```python
from build123d import *

# Parameters (mm, degrees)
BASPROSKE_W     = 100
BASPROSKE_H     = 56
TOOTHCUT_DEPTH  = 128.561749753
TEETHCUTS_COUNT = 12
TEETHCUTS_ANGLE = 330
BORSKE_R        = 20
BORE_DEPTH      = 100.0000508
SCALE1_SCALE    = 0.25


with BuildPart() as part:
    # BasProSke → Base-Revolve (revolve)
    with BuildSketch(Plane(origin=(0, 0, 0), x_dir=(1, 0, 0), z_dir=(0, 1, 0)), mode=Mode.PRIVATE) as base_revolve_sk:
        with Locations((50, 28)):
            Rectangle(BASPROSKE_W, BASPROSKE_H)
    revolve(base_revolve_sk.sketch.rotate(Axis((-10, 0, 0), (1, 0, 0)), 180), axis=Axis((-10, 0, 0), (1, 0, 0)))

    # TooCutSke → ToothCut (cut, through all)
    with BuildSketch(Plane(origin=(0, 0, 0), x_dir=(0, 0, -1), z_dir=(1, 0, 0))):
        with BuildLine():
            ThreePointArc((4.429508858, 37.739945049), (0, 37.999), (-4.429508858, 37.739945049))
            ThreePointArc((-4.429508858, 37.739945049), (-6.560078122, 47.242513828), (-13.078840191, 54.477420868))
            ThreePointArc((-13.078840191, 54.477420868), (0, 56.0254), (13.078840191, 54.477420868))
            ThreePointArc((13.078840191, 54.477420868), (6.560078122, 47.242513828), (4.429508858, 37.739945049))
        make_face()
    toothcut = extrude(amount=TOOTHCUT_DEPTH, mode=Mode.SUBTRACT)

    # TeethCuts: ToothCut ×12 about axis
    teethcuts_axis = Axis((-10, 0, 0), (1, 0, 0))
    for i in range(1, TEETHCUTS_COUNT):
        add(toothcut.rotate(teethcuts_axis, i * TEETHCUTS_ANGLE / (TEETHCUTS_COUNT - 1)), mode=Mode.SUBTRACT)

    # BorSke → Bore (cut, symmetric)
    with BuildSketch(Plane(origin=(0, 0, 0), x_dir=(0, 0, -1), z_dir=(1, 0, 0))):
        with Locations(Location((0, 0, 0), (0, 0, 180))):
            Circle(BORSKE_R)
    extrude(amount=BORE_DEPTH, both=True, mode=Mode.SUBTRACT)


with BuildPart() as part_1:
    # Scale1: scaled about (50, 0, 0)
    add(part.part.scale(SCALE1_SCALE).moved(Location((37.5, 0, 0))))


solid = part_1.part
```
The model under review builds one solid part; all positions refer to its coordinate system, in mm. A direction names the side the tool comes from. Round coordinates to 2 decimals unless told otherwise and drop trailing zeros. Loops run counter-clockwise (first coordinate to the right, second up) from the corner with the lowest first, then second, coordinate; pieces in that order, holes last. Notation, with made-up numbers: (-30.5, 59.25) -> (-7.5, 59.25) arc R18 cw to (-7.5, 82.25) -> close; hole circle Ø3 at (3.25, -2). An arc over 180 degrees is marked (long way). Answer as a JSON object with one key per item and string values. Group by question number.
1) Mouldability with a two-part tool opening along Z and no side actions: class faces 1 (the face through (49.825, 4.486, -11.078)), 2 (the face through (62.5, 0, -6)) as released by +Z, released by -Z, zero draft, split by the parting line, or undercut.
2) For line 1 (Y direction, x = 57.25, z = -4); line 2 (Y direction, x = 55.5, z = 0); line 3 (Y direction, x = 46.5, z = 8.75), list the stretches that pass through material, from the lowest coordinate up. Write a range as [from, to].
3) For pin 1 Ø2 at (x, y) = (51, -9.5) entering from +Z; pin 2 Ø5 at (x, z) = (48.5, -3.5) entering from +Y; pin 3 Ø1 at (x, y) = (59, -10.5) entering from -Z; pin 4 Ø10 at (x, y) = (43.5, 5) entering from +Z, all flat-tipped, find the tip position at first contact; note any pin that passes through.
4) We need section C-C on z = 6.5. Write out the cut boundary in (x, y).
5) We need section A-A on y = 0. Write out the cut boundary in (x, z).
6) For faces 3 (the face through (37.5, 0, -6)), 4 (the face through (49.825, 11.078, 4.486)), list the 3-axis set-ups (+Z, -Z, +X, -X, +Y, -Y) from which the entire face can be reached by the end or side of a thin tool; tool diameter is ignored.
Result set:
{
 "1": {"face 1": "undercut", "face 2": "zero draft"},
 "2": {"line 1": "[-13.39, -9.16], [-8.62, -3], [3, 8.62], [9.16, 13.39]", "line 2": "[-9.5, -5], [5, 9.5]", "line 3": "[-10.02, -6.51], [-3.77, 3.77], [6.51, 10.02]"},
 "3": {"pin 1": "z = 10.16", "pin 2": "y = 13.61", "pin 3": "z = -9.8", "pin 4": "z = 13.61"},
 "4": {"outline": "(37.5, -8.74) -> (62.5, -8.74) -> (62.5, 8.74) -> (37.5, 8.74) -> close"},
 "5": {"outline": "(37.5, -9.5) -> (62.5, -9.5) -> (62.5, -5) -> (37.5, -5) -> close; (37.5, 5) -> (62.5, 5) -> (62.5, 9.5) -> (37.5, 9.5) -> close"},
 "6": {"face 3": "+Z, -Z, -X, +Y, -Y", "face 4": "+X, -X"}
}
